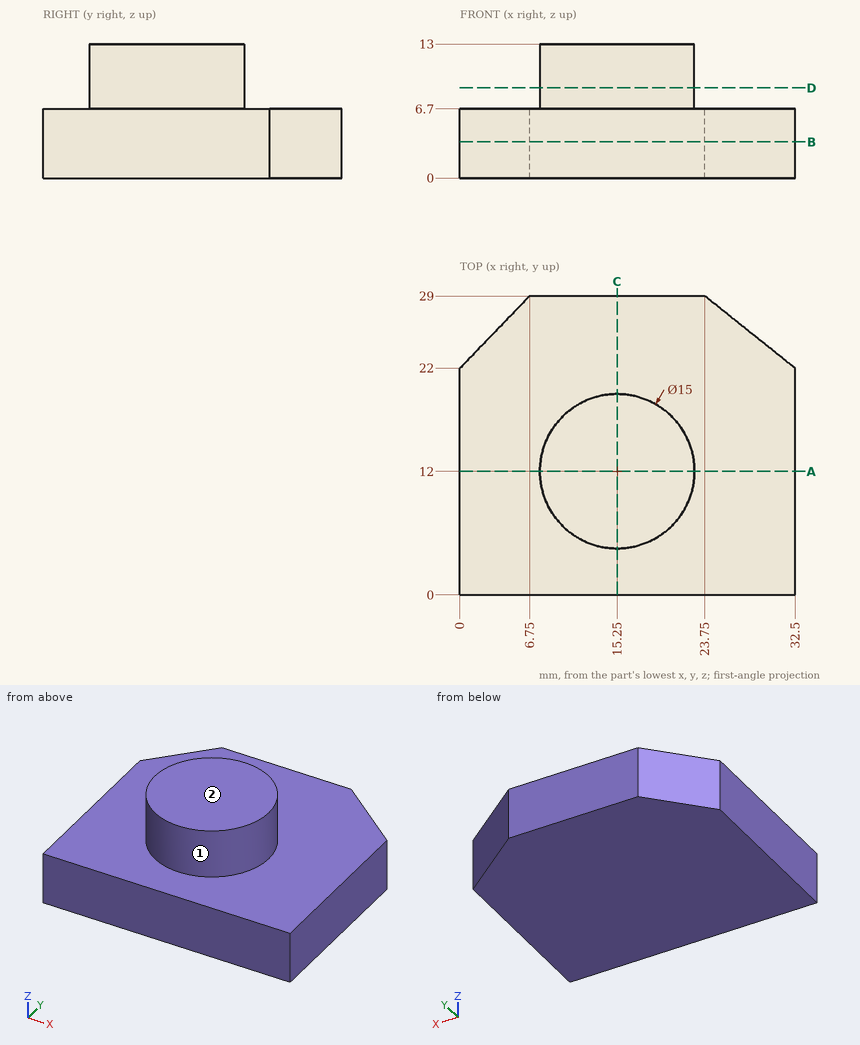
Geometry check sheet. Reference: drawing and pictorial views, mm from the part's lowest x, y, z. A direction names the side the tool comes from. Give positions to 0.01 mm unless a question says otherwise; leave off trailing zeros. Write each loop counter-clockwise with the first axis right and the second up, starting at its lowest first coordinate (ties: lowest second). Pieces come first, ordered by that corner, then holes.
Item 1: Scan lines: L1, parallel to Z at x = 28, y = 19; L2, parallel to Y at x = 26, z = 4; L3, parallel to Y at x = 27, z = 4.5. Record each from-to range of solid material in increasing order.
Item 2: Gauge pin test, flat ends, axial feed: pin 1 (1.5 mm diameter, centred on y = 13.5, z = 8.5, fed in from -X); pin 2 (4 mm diameter, centred on x = 20.5, y = 21, fed in from +Z); pin 3 (2 mm diameter, centred on y = 15, z = 9.5, fed in from +X); pin 4 (6 mm diameter, centred on x = 11.5, y = 8, fed in from -Z). Record the tip position at first contact, or that the pin passes through.
Item 3: Access from +Z, -Z, +X, -X, +Y, -Y to the whole of each face (thin tool, end or side, straight path). Record for the marked faces 1 and 2.
Item 4: Cross-section at D-D (z = 8.75). Enter the section's corners in (x, y), and give its area (3 significant figures).
Item 5: Cross-section at C-C (x = 15.25). Enter the section's corners in (y, z), and give its area (3 significant figures).
Item 6: Cross-section at A-A (y = 12). Enter the section's corners in (x, z).
Item 7: Cross-section at B-B (z = 3.5). Enter the section's corners in (x, y), and give its area (3 significant figures).
Report:
1. L1: z = 0 to 6.7
1. L2: y = 0 to 27.2
1. L3: y = 0 to 26.4
2. pin 1: stops at x = 7.79
2. pin 2: stops at z = 6.7
2. pin 3: stops at x = 22.48
2. pin 4: stops at z = 0
3. face 1: +Z
3. face 2: +Z, +X, -X, +Y, -Y
4. outline: circle Ø15 at (15.25, 12)
4. area: 177 mm2
5. outline: (0, 0) - (29, 0) - (29, 6.7) - (19.5, 6.7) - (19.5, 13) - (4.5, 13) - (4.5, 6.7) - (0, 6.7) - close
5. area: 289 mm2
6. outline: (0, 0) - (32.5, 0) - (32.5, 6.7) - (22.75, 6.7) - (22.75, 13) - (7.75, 13) - (7.75, 6.7) - (0, 6.7) - close
7. outline: (0, 0) - (32.5, 0) - (32.5, 22) - (23.75, 29) - (6.75, 29) - (0, 22) - close
7. area: 888 mm2
